Part model, mm, in its own coordinate system. A direction names the side the tool comes from. Round coordinates to 2 decimals unless told otherwise and drop trailing zeros. Write each loop counter-clockwise with the first axis right and the second up, starting at its lowest first coordinate (ties: lowest second). Pieces come first, ordered by that corner, then holes.
from build123d import *

# Parameters (mm, degrees)
SKETCH1_R           = 1.5
BOSS_EXTRUDE1_DEPTH = 2
BOSS_EXTRUDE2_DEPTH = 5


with BuildPart() as part:
    # Sketch1 → Boss-Extrude1 (new body)
    with BuildSketch(Plane.XY):
        with BuildLine():
            Line((0, 0), (10, 0))
            ThreePointArc((10, 0), (12.5, 2.5), (10, 5))
            Line((10, 5), (0, 5))
            ThreePointArc((0, 5), (-2.5, 2.5), (0, 0))
        make_face()
        with Locations((0, 2.5)):
            Circle(SKETCH1_R, mode=Mode.SUBTRACT)
        with Locations((10, 2.5)):
            Circle(SKETCH1_R, mode=Mode.SUBTRACT)
    extrude(amount=BOSS_EXTRUDE1_DEPTH)

    # Sketch2 → Boss-Extrude2 (add)
    with BuildSketch(Plane(origin=(0, 0, 0), x_dir=(1, 0, 0), z_dir=(0, 1, 0))):
        with BuildLine():
            Line((2.723714879, -2), (3.5, -2))
            Line((3.5, -2), (3.5, -7))
            Line((3.5, -7), (2.723714879, -7))
            add(Edge.make_bspline(
                [(2.723714879, -7), (2.623482732, -5.096496359), (2.626841272, -4.377777821), (2.43389568, -3.713843944), (2.176399926, -3.027645535), (1.933254484, -2)],
                knots=[0, 0, 0, 0, 0.37067554, 0.47067554, 1, 1, 1, 1], degree=3))
            Line((1.933254484, -2), (2.723714879, -2))
        make_face()
        with BuildLine():
            Line((8.066745516, -2), (7.276285121, -2))
            Line((7.276285121, -2), (6.5, -2))
            Line((6.5, -2), (6.5, -7))
            Line((6.5, -7), (7.276285121, -7))
            add(Edge.make_bspline(
                [(7.276285121, -7), (7.376517268, -5.096496359), (7.373158728, -4.377777821), (7.56610432, -3.713843944), (7.823600074, -3.027645535), (8.066745516, -2)],
                knots=[0, 0, 0, 0, 0.37067554, 0.47067554, 1, 1, 1, 1], degree=3))
        make_face()
    extrude(amount=BOSS_EXTRUDE2_DEPTH)


solid = part.part
Q1. Tool access for faces 1 (the flat face through (5, 5, 1)), 2 (the flat face through (11, 1, 2)), 3 (the flat face through (5, 3, 2)), 4 (the flat face through (-1, 4, 2)), 5 (the cylindrical face through (-2.5, 2.6, 1)): list every direction of +Z, -Z, +X, -X, +Y, -Y with a clear straight run to the whole face (end or side of a thin tool).
Q2. Two-plate mould, pull along Y, no slides. Class faces 6 (the cylindrical face through (0, 1, 1)), 7 (the cylindrical face through (8.8, 1.6, 1)), 8 (the cylindrical face through (12.5, 2.4, 1)), 9 (the flat face through (6.5, 2, 4)): released by +Y, released by -Y, zero draft, split by the parting line, or undercut.
Q3. Saw through at B-B, the plane z = 1. Write the cut outline in (x, y).
Q4. Wall check: line 1 (Y direction, x = 10, z = 0.65); line 2 (Z direction, x = 11.5, y = 2); line 3 (X direction, y = 4.55, z = 4.75). Give the ranges that are in metal, low to high.
Q5. Saw through at C-C, the plane y = 2.5. Give the number of separate pieces and of enclosed holes in the cut face, and give its area (3 significant figures).
Q6. Drop flat-ended pins along their axis: P1, Ø1.5, axis at y = 2.5, z = 4.5, coming from the -X side; P2, Ø2, axis at x = 0.5, z = 5.5, coming from the -Y side; P3, Ø1.5, axis at y = 3.5, z = 4.5, coming from the +X side. Give the stop position or say it passes through.
Q7. Saw through at A-A, the plane x = 9.5. Write the cut outline in (y, z).
Computed:
1. face 1: +Z, -Z, +X, -X, +Y
1. face 2: +Z, +X, +Y, -Y
1. face 3: +Z, +Y, -Y
1. face 4: +Z, -X, +Y, -Y
1. face 5: +Z, -Z, -X
2. face 6: undercut
2. face 7: undercut
2. face 8: split by the parting line
2. face 9: zero draft
3. outline: (0, 0) - (10, 0) arc R2.5 ccw to (10, 5) - (0, 5) arc R2.5 ccw to start; hole circle Ø3 at (0, 2.5); hole circle Ø3 at (10, 2.5)
4. line 1: y = 0 to 1, 4 to 5
4. line 2: z = 0 to 2
4. line 3: x = 2.62 to 3.5, 6.5 to 7.38
5. separate pieces: 3
5. enclosed holes: 0
5. area: 28.3 mm2
6. P1: stops at x = 2.44
6. P2: passes through
6. P3: stops at x = 7.56
7. outline: (0, 0) - (1.09, 0) - (1.09, 2) - (0, 2) - close; (3.91, 0) - (5, 0) - (5, 2) - (3.91, 2) - close
